The listing builds one solid part. Answer for the finished solid, in the listing's coordinates (mm). A direction names the side the tool comes from. Give positions to 0.01 mm unless a question says otherwise; leave off trailing zeros. Loops run counter-clockwise (first coordinate to the right, second up) from the corner with the lowest first, then second, coordinate; pieces in that order, holes last.
Item 1: Section D-D, the plane y = 2.4 is taken. Give the vertices of the cut face in (x, z).
Item 2: Section A-A, the plane z = 0 is taken. Give the vertices of the cut face in (x, y), and give its area (3 significant figures).
Item 3: Section B-B, the plane y = 1.15 is taken. Give the vertices of the cut face in (x, z), and give its area (3 significant figures).
Item 4: Consider line 1 along X through (y, z) = (1.25, 0); line 2 along Y through (x, z) = (2, 5.75). Determine where each line is inside the solid, lowest interval first.
Item 5: A tool of negligible diameter and unlimited length cuts with its end or side. For faces 5 (the face through (-0.75, 3.4, -5.7)), 6 (the face through (0, 5.85, 0)), from which of +Z, -Z, +X, -X, +Y, -Y can it reach the whole face along a straight path? Write none if from no direction.
Item 6: The mould has two halves that part along Z. Classify faces 1 (the face through (0, 1.85, 0)), 2 (the face through (-1.08, 0.91, 4.88)), 3 (the face through (-5.158, 0.74, 3.955)), 4 (the face through (2, 0, 5)): pulls with the +Z half, pulls with the -Z half, needs draft (parallel to the pull), parting line crosses it, or undercut.
Item 7: Section C-C, the plane x = 0 is taken. Give the vertices of the cut face in (y, z), and give its area (3 significant figures).
from build123d import *

# Parameters (mm, degrees)
SKETCH1_R           = 6.5
SKETCH1_R_2         = 5
BOSS_EXTRUDE1_DEPTH = 1.5
SKETCH2_R           = 5.75
SKETCH2_R_2         = 5
BOSS_EXTRUDE2_DEPTH = 4.35
FILLET1_R           = 0.5
SKETCH3_R           = 5
BOSS_EXTRUDE3_DEPTH = 4


with BuildPart() as part:
    # Sketch1 → Boss-Extrude1 (new body)
    with BuildSketch(Plane(origin=(0, 0, 0), x_dir=(1, 0, 0), z_dir=(0, 1, 0))):
        Circle(SKETCH1_R)
        Circle(SKETCH1_R_2, mode=Mode.SUBTRACT)
    extrude(amount=BOSS_EXTRUDE1_DEPTH)

    # Sketch2 → Boss-Extrude2 (add)
    with BuildSketch(Plane(origin=(0, 1.5, 0), x_dir=(1, 0, 0), z_dir=(0, 1, 0))):
        Circle(SKETCH2_R)
        Circle(SKETCH2_R_2, mode=Mode.SUBTRACT)
    extrude(amount=BOSS_EXTRUDE2_DEPTH)

    # Fillet1
    fillet1_edges = [part.edges().sort_by_distance(p)[0] for p in [
        (-5.75, 5.85, 0),
    ]]
    fillet(fillet1_edges, radius=FILLET1_R)

    # Sketch3 → Boss-Extrude3 (add)
    with BuildSketch(Plane(origin=(0, 5.85, 0), x_dir=(1, 0, 0), z_dir=(0, 1, 0))):
        Circle(SKETCH3_R)
    extrude(amount=-BOSS_EXTRUDE3_DEPTH)


solid = part.part
Worked answers:
1. outline: circle Ø11.5 at (0, 0)
2. outline: (-6.5, 0) - (-5, 0) - (-5, 1.85) - (5, 1.85) - (5, 0) - (6.5, 0) - (6.5, 1.5) - (5.75, 1.5) - (5.75, 5.35) arc R0.5 ccw to (5.25, 5.85) - (-5.25, 5.85) arc R0.5 ccw to (-5.75, 5.35) - (-5.75, 1.5) - (-6.5, 1.5) - close
2. area: 50.9 mm2
3. outline: circle Ø13 at (0, 0); hole circle Ø10 at (0, 0)
3. area: 54.2 mm2
4. line 1: x = -6.5 to -5, 5 to 6.5
4. line 2: y = 0 to 1.5
5. face 5: +Y
5. face 6: +Z, -Z, +X, -X, +Y
6. face 1: undercut
6. face 2: undercut
6. face 3: parting line crosses it
6. face 4: needs draft
7. outline: (0, -6.5) - (1.5, -6.5) - (1.5, -5.75) - (5.35, -5.75) arc R0.5 ccw to (5.85, -5.25) - (5.85, 5.25) arc R0.5 ccw to (5.35, 5.75) - (1.5, 5.75) - (1.5, 6.5) - (0, 6.5) - (0, 5) - (1.85, 5) - (1.85, -5) - (0, -5) - close
7. area: 50.9 mm2
